Build history of the part. All positions in model axes, mm. A direction names the side the tool comes from. Give positions to 0.01 mm unless a question says otherwise; leave off trailing zeros. Write each loop counter-clockwise with the first axis right and the second up, starting at its lowest first coordinate (ties: lowest second). Pieces come first, ordered by that corner, then holes.
from build123d import *

# Parameters (mm, degrees)
SKETCH1_W                        = 38.1
SKETCH1_H                        = 43.18
BOSS_EXTRUDE1_DEPTH              = 12.7
SKETCH3_R                        = 11
CUT_EXTRUDE1_DEPTH               = 13.7
F_17_64_0_26563_DIAMETER_HOLE1_D = 6.747002
F_1_4_20_TAPPED_HOLE2_D          = 5.1054
F_1_4_20_TAPPED_HOLE2_DEPTH      = 12.7
F_1_4_20_TAPPED_HOLE2_TIP        = 1.533816902


with BuildPart() as part:
    # Sketch1 → Boss-Extrude1 (new body)
    with BuildSketch(Plane.XY):
        with Locations((19.05, 21.59)):
            Rectangle(SKETCH1_W, SKETCH1_H)
    extrude(amount=-BOSS_EXTRUDE1_DEPTH)

    # Sketch3 → Cut-Extrude1 (cut, through all)
    with BuildSketch(Plane.XY):
        with Locations((19.05, 15.24)):
            Circle(SKETCH3_R)
    extrude(amount=-CUT_EXTRUDE1_DEPTH, mode=Mode.SUBTRACT)

    # 17/64 (0.26563) Diameter Hole1 (through all)
    with Locations(Plane(origin=(29.21, 36.83, 0), x_dir=(1, 0, 0), z_dir=(0, 0, 1))):
        with Locations((0, 0), (-20.32, 0)):
            Hole(F_17_64_0_26563_DIAMETER_HOLE1_D / 2)

    # 1/4-20 Tapped Hole2
    with Locations(Plane(origin=(0, 27.94, -6.35), x_dir=(0, 0, -1), z_dir=(-1, 0, 0))):
        with Locations((0, 0)):
            Hole(F_1_4_20_TAPPED_HOLE2_D / 2, depth=F_1_4_20_TAPPED_HOLE2_DEPTH)
            with Locations((0, 0, -(F_1_4_20_TAPPED_HOLE2_DEPTH + F_1_4_20_TAPPED_HOLE2_TIP / 2))):  # 118° drill point
                Cone(0, F_1_4_20_TAPPED_HOLE2_D / 2, F_1_4_20_TAPPED_HOLE2_TIP, mode=Mode.SUBTRACT)


solid = part.part
(1) 3-axis set-ups, long thin cutter, end or side, ignore diameter. For faces 4 (the face through (6.439, 30.432, -6.903)), 5 (the face through (0, 21, -6)): which of +Z, -Z, +X, -X, +Y, -Y reach the whole face in a straight line?
(2) Saw through at D-D, the plane y = 38.5. List the corners of the cut face in (x, z).
(3) Saw through at B-B, the plane z = -1. List the corners of the cut face in (x, y), plus the area to 3 significant figures.
(4) Saw through at C-C, the plane y = 11. List the corners of the cut face in (x, z), plus the area to 3 significant figures.
(5) Saw through at A-A, the plane x = 19.05. List the corners of the cut face in (y, z).
(6) Probe line 1 (X direction, y = 37, z = -9.5); line 2 (Y direction, x = 27, z = -9.25); line 3 (Y direction, x = 29.21, z = -8.75). List the from-to ranges inside material, lowest first.
(7) Drop a flat-ended pin along its axis: pin 1 (5.5 mm diameter, centred on x = 8.89, y = 36.83, fed in from -Z). Give the stop position or say it passes through.
(8) Mould opens along Y. For faces 1 (the face through (19, 0, -6)), 2 (the face through (19, 27, -12.7)), 3 (the face through (24.126, 5.481, -6.261)) say: +Y half, -Y half, draft (parallel to the pull), parting line (faces both ways), or undercut.
Computed values:
1. face 4: -X
1. face 5: +Z, -Z, -X, +Y, -Y
2. outline: (0, -12.7) - (5.96, -12.7) - (5.96, 0) - (0, 0) - close; (11.82, -12.7) - (26.28, -12.7) - (26.28, 0) - (11.82, 0) - close; (32.14, -12.7) - (38.1, -12.7) - (38.1, 0) - (32.14, 0) - close
3. outline: (0, 0) - (38.1, 0) - (38.1, 43.18) - (0, 43.18) - close; hole circle Ø6.75 at (8.89, 36.83); hole circle Ø22 at (19.05, 15.24); hole circle Ø6.75 at (29.21, 36.83)
3. area: 1,190 mm2
4. outline: (0, -12.7) - (8.9, -12.7) - (8.9, 0) - (0, 0) - close; (29.2, -12.7) - (38.1, -12.7) - (38.1, 0) - (29.2, 0) - close
4. area: 226 mm2
5. outline: (0, -12.7) - (4.24, -12.7) - (4.24, 0) - (0, 0) - close; (26.24, -12.7) - (43.18, -12.7) - (43.18, 0) - (26.24, 0) - close
6. line 1: x = 0 to 5.52, 12.26 to 25.84, 32.58 to 38.1
6. line 2: y = 0 to 7.64, 22.84 to 34.28, 39.38 to 43.18
6. line 3: y = 0 to 11.02, 19.46 to 33.46, 40.2 to 43.18
7. pin 1: passes through
8. face 1: -Y half
8. face 2: draft
8. face 3: undercut
